from build123d import *

# Parameters (mm, degrees)
SKETCH2_W           = 287
SKETCH2_H           = 65
BOSS_EXTRUDE1_DEPTH = 5
SKETCH4_W           = 5
SKETCH4_H           = 65
BOSS_EXTRUDE2_DEPTH = 25.5
SKETCH5_W           = 5
SKETCH5_H           = 65
BOSS_EXTRUDE3_DEPTH = 25.5
SKETCH6_W           = 5
SKETCH6_H           = 65
BOSS_EXTRUDE4_DEPTH = 25.5
SKETCH8_W           = 5
SKETCH8_H           = 65
BOSS_EXTRUDE5_DEPTH = 25.5
CUT_EXTRUDE1_REACH  = 299.556
SKETCH7_R           = 6.5
CUT_EXTRUDE2_REACH  = 299.556
SKETCH9_R           = 6.5
CUT_EXTRUDE3_REACH  = 223.403
SKETCH11_R          = 4.5
CUT_EXTRUDE4_REACH  = 223.403
SKETCH10_R          = 4.5
SKETCH14_W          = 1
SKETCH14_H          = 25.5
BOSS_EXTRUDE6_DEPTH = 1
CUT_EXTRUDE6_REACH  = 218.736
SKETCH15_R          = 2


with BuildPart() as part:
    # Sketch2 → Boss-Extrude1 (new body)
    with BuildSketch(Plane(origin=(0, 0, 0), x_dir=(1, 0, 0), z_dir=(0, 1, 0))):
        with Locations((100.827281974, 41.798134807)):
            Rectangle(SKETCH2_W, SKETCH2_H)
    extrude(amount=BOSS_EXTRUDE1_DEPTH)

    # Sketch4 → Boss-Extrude2 (add)
    with BuildSketch(Plane.XZ):
        with Locations((-40.172718026, -41.798134807)):
            Rectangle(SKETCH4_W, SKETCH4_H)
    extrude(amount=BOSS_EXTRUDE2_DEPTH)

    # Sketch5 → Boss-Extrude3 (add)
    with BuildSketch(Plane.XZ):
        with Locations((39.827281974, -41.798134807)):
            Rectangle(SKETCH5_W, SKETCH5_H)
    extrude(amount=BOSS_EXTRUDE3_DEPTH)

    # Sketch6 → Boss-Extrude4 (add)
    with BuildSketch(Plane.XZ):
        with Locations((241.827281974, -41.798134807)):
            Rectangle(SKETCH6_W, SKETCH6_H)
    extrude(amount=BOSS_EXTRUDE4_DEPTH)

    # Sketch8 → Boss-Extrude5 (add)
    with BuildSketch(Plane.XZ):
        with Locations((161.827281974, -41.798134807)):
            Rectangle(SKETCH8_W, SKETCH8_H)
    extrude(amount=BOSS_EXTRUDE5_DEPTH)

    # Sketch7 → Cut-Extrude1 (cut, up to next)
    with BuildSketch(Plane.ZY.offset(42.672718026), mode=Mode.PRIVATE) as cut_extrude1_sk1:
        with Locations((-30.964801474, -12.75)):
            Circle(SKETCH7_R)
    cut_extrude1_tool1 = extrude(cut_extrude1_sk1.sketch, amount=-CUT_EXTRUDE1_REACH, mode=Mode.PRIVATE) & part.part
    add(cut_extrude1_tool1.solids().sort_by_distance((-42.672718, -12.75, -30.964801))[0], mode=Mode.SUBTRACT)

    # Sketch9 → Cut-Extrude2 (cut, up to next)
    with BuildSketch(Plane(origin=(244.327281974, 0, 0), x_dir=(0, 0, -1), z_dir=(1, 0, 0)), mode=Mode.PRIVATE) as cut_extrude2_sk1:
        with Locations((52.631468141, -12.75)):
            Circle(SKETCH9_R)
    cut_extrude2_tool1 = extrude(cut_extrude2_sk1.sketch, amount=-CUT_EXTRUDE2_REACH, mode=Mode.PRIVATE) & part.part
    add(cut_extrude2_tool1.solids().sort_by_distance((244.327282, -12.75, -52.631468))[0], mode=Mode.SUBTRACT)

    # Sketch11 → Cut-Extrude3 (cut, up to next)
    with BuildSketch(Plane(origin=(164.327281974, 0, 0), x_dir=(0, 0, -1), z_dir=(1, 0, 0)), mode=Mode.PRIVATE) as cut_extrude3_sk1:
        with Locations((52.631468141, -12.75)):
            Circle(SKETCH11_R)
    cut_extrude3_tool1 = extrude(cut_extrude3_sk1.sketch, amount=-CUT_EXTRUDE3_REACH, mode=Mode.PRIVATE) & part.part
    add(cut_extrude3_tool1.solids().sort_by_distance((164.327282, -12.75, -52.631468))[0], mode=Mode.SUBTRACT)

    # Sketch10 → Cut-Extrude4 (cut, up to next)
    with BuildSketch(Plane.ZY.offset(-37.327281974), mode=Mode.PRIVATE) as cut_extrude4_sk1:
        with Locations((-30.964801474, -12.75)):
            Circle(SKETCH10_R)
    cut_extrude4_tool1 = extrude(cut_extrude4_sk1.sketch, amount=-CUT_EXTRUDE4_REACH, mode=Mode.PRIVATE) & part.part
    add(cut_extrude4_tool1.solids().sort_by_distance((37.327282, -12.75, -30.964801))[0], mode=Mode.SUBTRACT)

    # Sketch14 → Boss-Extrude6 (add)
    with BuildSketch(Plane.ZY.offset(-159.327281974)):
        with Locations((-15.468134807, -12.75)):
            Rectangle(SKETCH14_W, SKETCH14_H)
        with Locations((-46.468134807, -12.75)):
            Rectangle(SKETCH14_W, SKETCH14_H)
    extrude(amount=BOSS_EXTRUDE6_DEPTH)

    # Sketch15 → Cut-Extrude6 (cut, up to next)
    with BuildSketch(Plane.ZY.offset(-159.327281974), mode=Mode.PRIVATE) as cut_extrude6_sk1:
        with Locations((-20.968134807, -12.75)):
            Circle(SKETCH15_R)
    cut_extrude6_tool1 = extrude(cut_extrude6_sk1.sketch, amount=-CUT_EXTRUDE6_REACH, mode=Mode.PRIVATE) & part.part
    # Sketch15 → Cut-Extrude6 (cut, up to next)
    with BuildSketch(Plane.ZY.offset(-159.327281974), mode=Mode.PRIVATE) as cut_extrude6_sk2:
        with Locations((-40.968134807, -12.75)):
            Circle(SKETCH15_R)
    cut_extrude6_tool2 = extrude(cut_extrude6_sk2.sketch, amount=-CUT_EXTRUDE6_REACH, mode=Mode.PRIVATE) & part.part
    # Sketch15 → Cut-Extrude6 (cut, up to next)
    with BuildSketch(Plane.ZY.offset(-159.327281974), mode=Mode.PRIVATE) as cut_extrude6_sk3:
        with Locations((-30.968134807, -21.75)):
            Circle(SKETCH15_R)
    cut_extrude6_tool3 = extrude(cut_extrude6_sk3.sketch, amount=-CUT_EXTRUDE6_REACH, mode=Mode.PRIVATE) & part.part
    # Sketch15 → Cut-Extrude6 (cut, up to next)
    with BuildSketch(Plane.ZY.offset(-159.327281974), mode=Mode.PRIVATE) as cut_extrude6_sk4:
        with Locations((-30.968134807, -3.75)):
            Circle(SKETCH15_R)
    cut_extrude6_tool4 = extrude(cut_extrude6_sk4.sketch, amount=-CUT_EXTRUDE6_REACH, mode=Mode.PRIVATE) & part.part
    add(cut_extrude6_tool1.solids().sort_by_distance((159.327282, -12.75, -20.968135))[0], mode=Mode.SUBTRACT)
    add(cut_extrude6_tool2.solids().sort_by_distance((159.327282, -12.75, -40.968135))[0], mode=Mode.SUBTRACT)
    add(cut_extrude6_tool3.solids().sort_by_distance((159.327282, -21.75, -30.968135))[0], mode=Mode.SUBTRACT)
    add(cut_extrude6_tool4.solids().sort_by_distance((159.327282, -3.75, -30.968135))[0], mode=Mode.SUBTRACT)


solid = part.part
Work out the finished part from the listing and answer in its coordinate system (mm). A direction names the side the tool comes from. Give positions to 0.01 mm unless a question says otherwise; leave off trailing zeros. Loops run counter-clockwise (first coordinate to the right, second up) from the corner with the lowest first, then second, coordinate; pieces in that order, holes last. Notation, with made-up numbers: (-10.5, -17) -> (42.5, -17) arc R22 cw to (42.5, 6) -> close; hole circle Ø10 at (-12, 6). An arc over 180 degrees is marked (long way). Use a Markdown table: item, result. Add a question column.
1. Section A-A on z = -62 is taken. Determine the outline of the cut face in (x, y), and give its area (4 significant figures).
2. Flat-ended cylindrical pins translate along their axes: pin 1 Ø5 at (y, z) = (-10.5, -54) entering from +X; pin 2 Ø2 at (x, z) = (155.5, -51) entering from -Y; pin 3 Ø8 at (y, z) = (-12.75, -30.96) entering from -X. Find the tip coordinate at first contact, or state that the pin passes through.
3. Find the intervals of material crossed by probe 1 along X at (y, z) = (-19.5, -45.5); probe 2 along X at (y, z) = (-18.5, -46.5); probe 3 along X at (y, z) = (-14.5, -36), in increasing order.
4. Determine the mould class of faces 1 (the flat face through (99, 5, -42)), 2 (the cylindrical face through (39.79, -12.55, -35.46)), 3 (the flat face through (90, 2, -74.298)), 4 (the flat face through (242, -25.5, -41)) for opening direction Y: released by +Y, released by -Y, zero draft, split by the parting line, or undercut.
5. For faces 5 (the cylindrical face through (-40.21, -12.46, -37.46)), 6 (the flat face through (-1, 0, -42)), 7 (the flat face through (159.327, -13, -31)), determine the directions among +Z, -Z, +X, -X, +Y, -Y from which every point of the face is accessible in a straight line to the end or side of a thin tool.
6. Section B-B on x = 85 is taken. Determine the outline of the cut face in (y, z).
Results below:
| question | item | result |
|---|---|---|
| 1 | outline | (-42.67, -25.5) -> (-37.67, -25.5) -> (-37.67, 0) -> (37.33, 0) -> (37.33, -25.5) -> (42.33, -25.5) -> (42.33, 0) -> (159.33, 0) -> (159.33, -25.5) -> (164.33, -25.5) -> (164.33, 0) -> (239.33, 0) -> (239.33, -25.5) -> (244.33, -25.5) -> (244.33, 5) -> (-42.67, 5) -> close |
| 1 | area | 1,945 mm^2 |
| 2 | pin 1 | stops at x = 164.33 |
| 2 | pin 2 | stops at y = 0 |
| 2 | pin 3 | stops at x = 159.33 |
| 3 | probe 1 | x = -42.67 to -37.67, 37.33 to 42.33, 159.33 to 164.33, 239.33 to 244.33 |
| 3 | probe 2 | x = -42.67 to -37.67, 37.33 to 42.33, 158.33 to 164.33, 239.33 to 244.33 |
| 3 | probe 3 | x = 37.33 to 42.33, 159.33 to 164.33, 239.33 to 244.33 |
| 4 | face 1 | released by +Y |
| 4 | face 2 | undercut |
| 4 | face 3 | zero draft |
| 4 | face 4 | released by -Y |
| 5 | face 5 | -X |
| 5 | face 6 | +Z, -Z, -Y |
| 5 | face 7 | -Y |
| 6 | outline | (0, -74.3) -> (5, -74.3) -> (5, -9.3) -> (0, -9.3) -> close |
